The model under review builds one solid part; all positions refer to its coordinate system, in mm. A direction names the side the tool comes from. Coordinates: 2 decimals unless noted, no trailing zeros. Loops run counter-clockwise (first coordinate to the right, second up) from the corner with the lowest first, then second, coordinate; pieces in that order, holes last. Notation, with made-up numbers: M 15,39.25 L 61,39.25 A17 cw 61,48.25 Z; hole C -13.75,14 d9. An arc over 180 degrees is marked long. Return JSON: item names as keys, results as strings.
```python
from build123d import *

# Parameters (mm, degrees)
SKETCH_1_R            = 11
EXTRUDE_1_DEPTH       = 10
CUT_EXTRUDE_1_DEPTH   = 11
FILLET_1_R            = 1.5
M4X0_71_D             = 3.3
M4X0_71_DEPTH         = 5
M4X0_71_TIP           = 0.991420021
HOLE_WIZARD_M41_D     = 4.5
HOLE_WIZARD_M41_DEPTH = 6.466619964
M4X0_72_D             = 3.3
FILLET_2_R            = 3
CUT_EXTRUDE_2_DEPTH   = 11
FILLET_3_R            = 2
FILLET_5_R            = 8


with BuildPart() as part:
    # Эскиз1 → Бобышка-Вытянуть1 (new body)
    with BuildSketch(Plane.XY):
        with BuildLine():
            Line((-31.75, -12), (-9.910576673, 9.888400781))
            ThreePointArc((-9.910576673, 9.888400781), (0, 14), (9.910576673, 9.888400781))
            Line((9.910576673, 9.888400781), (31.75, -12))
            Line((31.75, -12), (31.75, -17))
            Line((31.75, -17), (-31.75, -17))
            Line((-31.75, -17), (-31.75, -12))
        make_face()
        Circle(SKETCH_1_R, mode=Mode.SUBTRACT)
    extrude(amount=EXTRUDE_1_DEPTH)

    # Эскиз2 → Вырез-Вытянуть1 (cut, through all)
    with BuildSketch(Plane.XY.offset(10)):
        Polygon((10.994327356, -0.353222306), (18.623994631, -8), (31.75, -8), (31.75, -12), (16.964515327, -12), (9.858995646, -4.878545362), align=None)
    extrude(amount=-CUT_EXTRUDE_1_DEPTH, mode=Mode.SUBTRACT)

    # Скругление1
    fillet_1_edges = [part.edges().sort_by_distance(p)[0] for p in [
        (27.758950394, -8, 5),
        (18.623994631, -8, 5),
        (9.858995646, -4.878545362, 5),
        (10.994327356, -0.353222306, 5),
        (16.964515327, -12, 5),
    ]]
    fillet(fillet_1_edges, radius=FILLET_1_R)

    # Отверстие обработанное метчиком M4x0.71
    with Locations(Plane(origin=(0, -17, 0), x_dir=(-1, 0, 0), z_dir=(0, -1, 0))):
        with Locations((26.75, -5), (-26.75, -5)):
            Hole(M4X0_71_D / 2, depth=M4X0_71_DEPTH)
            with Locations((0, 0, -(M4X0_71_DEPTH + M4X0_71_TIP / 2))):  # 118° drill point
                Cone(0, M4X0_71_D / 2, M4X0_71_TIP, mode=Mode.SUBTRACT)

    # Отверстие с зазором M41
    with Locations(Plane(origin=(9.910576673, 9.888400781, 0), x_dir=(0, 0, -1), z_dir=(0.707898334, 0.706314342, 0))):
        with Locations((-5, -15.654139496)):
            Hole(HOLE_WIZARD_M41_D / 2, depth=HOLE_WIZARD_M41_DEPTH)

    # Отверстие обработанное метчиком M4x0.72 (through all)
    with Locations(Plane(origin=(2.50127384, 2.495676993, 0), x_dir=(0, 0, -1), z_dir=(0.707898334, 0.706314342, 0))):
        with Locations((-5, -15.654139496)):
            Hole(M4X0_72_D / 2)

    # Скругление2
    fillet_2_edges = [part.edges().sort_by_distance(p)[0] for p in [
        (31.75, -12, 5),
    ]]
    fillet(fillet_2_edges, radius=FILLET_2_R)

    # Эскиз11 → Вырез-Вытянуть2 (cut, through all)
    with BuildSketch(Plane.XY.offset(10)):
        with BuildLine():
            Line((-13.9037433, 1.638878353), (-24.107110728, -8.587371317))
            ThreePointArc((-24.107110728, -8.587371317), (-24.53864421, -10.766401538), (-22.69131406, -12))
            Line((-22.69131406, -12), (-7.211102551, -12))
            ThreePointArc((-7.211102551, -12), (-12.568370201, -6.167339012), (-13.9037433, 1.638878353))
        make_face()
    extrude(amount=-CUT_EXTRUDE_2_DEPTH, mode=Mode.SUBTRACT)

    # Скругление3
    fillet_3_edges = [part.edges().sort_by_distance(p)[0] for p in [
        (-13.9037433, 1.638878353, 5),
        (-7.211102551, -12, 5),
    ]]
    fillet(fillet_3_edges, radius=FILLET_3_R)

    # Скругление5
    fillet_5_edges = [part.edges().sort_by_distance(p)[0] for p in [
        (-31.75, -12, 5),
    ]]
    fillet(fillet_5_edges, radius=FILLET_5_R)


solid = part.part
```
1. Insertion check: pin 1 Ø1 at (y, z) = (-2.5, 1.5) entering from +X; pin 2 Ø3 at (x, z) = (-26.75, 5) entering from +Y; pin 3 Ø4 at (x, z) = (8, 8.5) entering from +Y. Each pin has a flat end and moves straight along its axis. Give the tip position at first contact, or say it passes through.
Check values:
{"pin 1": "x = 22.77", "pin 2": "y = -5.49", "pin 3": "y = 12.65"}
2. Machinability: for faces 1 (the face through (22, -8, 5)), 2 (the face through (25.1, -14.46, 4.93)), 3 (the face through (-19.798, -0.022, 4.93)), 4 (the face through (-20.57, -5.04, 5.07)), which of the approach directions +Z, -Z, +X, -X, +Y, -Y give a long, thin tool a straight path to every point of the face, cutting with its end or side? Answer none if there is none.
Check values:
{"face 1": "+Z, -Z, +X", "face 2": "-Y", "face 3": "+Z, -Z, -X, +Y", "face 4": "+Z, -Z"}
3. To check wall thickness, follow line 1 (X direction, y = -1.5, z = 7.5); line 2 (Z direction, x = 26.75, y = -13.3); line 3 (X direction, y = -2, z = 7.5). State the ranges of each line that lie inside material, in increasing order.
Check values:
{"line 1": "-21.27 to -17.03, -14.4 to -10.9, 12.14 to 21.27", "line 2": "0 to 3.35, 6.65 to 10", "line 3": "-21.77 to -17.53, -13.99 to -10.82, 12.64 to 21.77"}
4. The part is to be moulded in two halves that separate along Z. For faces 5 (the face through (-2, -12, 0)), 6 (the face through (0, -17, 5)), 7 (the face through (18.169, -3.03, 7.146)), 8 (the face through (-28.4, -14.46, 4.93)), say which applies: released by +Z, released by -Z, zero draft, split by the parting line, or undercut.
Check values:
{"face 5": "released by -Z", "face 6": "zero draft", "face 7": "undercut", "face 8": "undercut"}
5. Add section B-B on z = 9.25. Give the boundary of the cut face in (x, y).
Check values:
{"outline": "M -31.75,-17 L 31.75,-17 L 31.75,-15 A3 ccw 28.75,-12 L 17.59,-12 A1.5 cw 16.52,-11.56 L 11.21,-6.24 A1.5 ccw 8.93,-6.42 A11 cw long 11,0.23 A1.5 ccw 11.44,-0.8 L 18.18,-7.56 A1.5 ccw 19.25,-8 L 24.14,-8 A1.5 ccw 25.21,-5.44 L 9.91,9.89 A14 ccw -9.91,9.89 L -29.41,-9.66 A8 ccw -31.75,-15.31 Z; hole M -24.11,-8.59 A2 ccw -22.69,-12 L -12.49,-12 A2 ccw -10.93,-8.75 A14 cw -13.75,-2.63 A2 ccw -17.13,-1.6 Z"}
6. Add section C-C on x = 0.5. Give the boundary of the cut face in (y, z).
Check values:
{"outline": "M -17,0 L -10.99,0 L -10.99,10 L -17,10 Z; M 10.99,0 L 13.99,0 L 13.99,10 L 10.99,10 Z"}
7. Add section A-A on x = 26.75. Give the boundary of the cut face in (y, z), plus the area to 3 significant figures.
Check values:
{"outline": "M -17,0 L -12,0 L -12,3.35 L -17,3.35 Z; M -17,6.65 L -12,6.65 L -12,10 L -17,10 Z", "area": "33.5 mm²"}
